```python
from build123d import *

# Parameters (mm, degrees)
SKETCH036_R           = 4.445
POCKET003_DEPTH       = 461.643083323
POLARPATTERN003_COUNT = 6
CHAMFER_SIZE          = 2.032
FILLET_R              = 3.175
FILLET001_R           = 0.79375
FILLET002_R           = 8.001


with BuildPart() as part:
    # Sketch035 → Revolution006 (revolve)
    with BuildSketch(Plane.XZ):
        Polygon((0, 78.5749), (-11.176, 78.5749), (-11.176, 53.1749), (-4.191, 40.4749), (-4.191, 33.4899), (-11.176, 18.2499), (-11.176, 16.7005), (-36.576, 16.7005), (-36.576, 12.7), (-8.9407358595, 12.7), (-8.9407358595, 18.2499), (-2.159, 33.0464146026), (-2.159, 40.9968329476), (-9.144, 53.6968329476), (-9.144, 76.5429), (0, 76.5429), align=None)
    revolve(axis=Axis((0, 0, 0), (1, 0, 0)))

    # Sketch036 → Pocket003 (cut, through all)
    with BuildSketch(Plane(origin=(-11.176, 0, 0), x_dir=(0, 0, -1), z_dir=(-1, 0, 0))):
        with Locations((-63.5, 0)):
            Circle(SKETCH036_R)
    pocket003 = extrude(amount=-POCKET003_DEPTH, mode=Mode.SUBTRACT)

    # PolarPattern003: Pocket003 ×6 about axis
    polarpattern003_axis = Axis((-11.176, 0, 0), (-1, 0, 0))
    for i in range(1, POLARPATTERN003_COUNT):
        add(pocket003.rotate(polarpattern003_axis, i * 360 / POLARPATTERN003_COUNT), mode=Mode.SUBTRACT)

    # Chamfer
    chamfer_edges = [part.edges().sort_by_distance(p)[0] for p in [
        (-36.576, 0, -16.7005),
    ]]
    chamfer(chamfer_edges, length=CHAMFER_SIZE)

    # Fillet
    fillet_edges = [part.edges().sort_by_distance(p)[0] for p in [
        (-11.176, 0, -78.5749),
    ]]
    fillet(fillet_edges, radius=FILLET_R)

    # Fillet001
    fillet001_edges = [part.edges().sort_by_distance(p)[0] for p in [
        (-9.144, 0, -76.5429),
    ]]
    fillet(fillet001_edges, radius=FILLET001_R)

    # Fillet002
    fillet002_edges = [part.edges().sort_by_distance(p)[0] for p in [
        (-2.159, 0, -33.046415),
        (-2.159, 0, -40.996833),
    ]]
    fillet(fillet002_edges, radius=FILLET002_R)


with BuildPart() as part_1:
    # Body011 placement: moved
    add(part.part.moved(Location((-320.04, 0, 0))))


solid = part_1.part
```
The listing builds one solid part. Answer for the finished solid, in the listing's coordinates (mm). A direction names the side the tool comes from. Coordinates: 2 decimals unless noted, no trailing zeros. Loops run counter-clockwise (first coordinate to the right, second up) from the corner with the lowest first, then second, coordinate; pieces in that order, holes last. Notation, with made-up numbers: M 74.5,89.25 L 115.5,89.25 A14 ccw 115.5,111.25 Z; hole C 51,23.25 d8. An arc over 180 degrees is marked long. Answer as a JSON object with one key per item and string values. Group by question number.
Item 1: Each of these flat-tipped pins is pushed along its axis until it touches: P1, Ø3, axis at x = -337, z = 10, coming from the +Y side; P2, Ø1, axis at y = 15, z = -3.5, coming from the -X side; P3, Ø5.5, axis at y = 54.99, z = -31.75, coming from the +X side; P4, Ø10, axis at y = -54.99, z = -31.75, coming from the +X side. Where does it stop, or does it pass through?
Item 2: Consider L1, parallel to Z at x = -322, y = 0; L2, parallel to Y at x = -329.7, z = -31.75; L3, parallel to Y at x = -329.5, z = 31. Determine where each line is inside the solid, lowest interval first.
Item 3: Section A-A (y = 0) is taken. Give the number of separate pieces and of enclosed holes in the cut face, and give its area (3 significant figures).
Item 4: Which of the six approach directions +Z, -Z, +X, -X, +Y, -Y give full straight-line access (tool end or side, diameter ignored) to faces 1 (the face through (-324.231, -30.2, -15.2)), 2 (the face through (-330.214, -51.245, 34.14)), 3 (the face through (-322.199, -32, 15))?
Item 5: Section B-B (x = -341) is taken. Write down the section's boundary in (y, z).
Item 6: Determine the mould class of faces 4 (the face through (-330.214, 50.585, -31.171)), 5 (the face through (-331.216, 15, 8)), 6 (the face through (-328.602, 18.623, -4.135)), 7 (the face through (-343.064, 16.303, -3.62)) for opening direction Z: +Z half, -Z half, draft (parallel to the pull), parting line (faces both ways), or undercut.
Solved:
{
 "1": {"P1": "stops at y = 14.38", "P2": "stops at x = -356.38", "P3": "passes through", "P4": "stops at x = -329.18"},
 "2": {"L1": "z = -78.57 to -76.54, 76.54 to 78.57", "L2": "y = -71.36 to -59.44, -50.55 to -39.17, 39.17 to 50.55, 59.44 to 71.36", "L3": "y = -71.81 to -59.37, -50.61 to -39.3, 39.3 to 50.61, 59.37 to 71.81"},
 "3": {"separate pieces": "4", "enclosed holes": "0", "area": "478 mm2"},
 "4": {"face 1": "-X", "face 2": "+X, -X", "face 3": "+X"},
 "5": {"outline": "C 0,0 d33.4; hole C 0,0 d25.4"},
 "6": {"face 4": "undercut", "face 5": "draft", "face 6": "undercut", "face 7": "parting line"}
}
